Autodesk Inventor part; units mm, degrees
ref_plane "YZ Plane" through (0, 0, 0) normal (1, 0, 0) x (0, 1, 0)
ref_plane "XZ Plane" through (0, 0, 0) normal (0, 1, 0) x (-1, 0, 0)
ref_plane "XY Plane" through (0, 0, 0) normal (0, 0, 1) x (1, 0, 0)
sketch "Skizze1" plane through (0, 0, 0) normal (0, 0, 1) x (1, 0, 0)
  line L0 (0, 0) -> (-67, 0)
  line L1 (-51, 5) -> (0, 5)
  line L2 (0, 5) -> (0, 0)
  line L3 (-51, 5) -> (-51, 2)
  line L4 (-51, 2) -> (-55, 2)
  line L5 (-55, 2) -> (-55, 0)
  line L6 (-56, 0) -> (-55, 0)
  dimension "d0" = 51
  dimension "d42" = 10
  dimension "d60" = 4
  dimension "d61" = 4
revolve "Umdrehung1" add sketch "Skizze1" angle 360 about axis through (0, 0, 0) along (-1, 0, 0)
sketch "Skizze3" plane through (0, 0, 0) normal (0, 1, 0) x (-1, 0, 0)
  line L0 (51, 5) -> (51, -5) construction
  line L1 (51, -5) -> (0, -5) construction
  line L2 (51, 5) -> (0, 5) construction
  line L3 (51, -5) -> (4, -5)
  line L4 (4, -5) -> (4, -3.5)
  line L5 (4, -3.5) -> (51, -3.5)
  line L6 (51, -3.5) -> (51, -5)
  line L7 (4, 5) -> (51, 5)
  line L8 (51, 5) -> (51, 3.5)
  line L9 (51, 3.5) -> (4, 3.5)
  line L10 (4, 3.5) -> (4, 5)
  line L11 (0, 5) -> (0, -5)
  point P0 (0, 0)
  dimension "d10" = 7
  dimension "d11" = 4
extrude "Extrusion1" cut sketch "Skizze3" along normal through all both and the other way through all
sketch "Skizze8" plane through (-4, -3.5707, 3.5) normal (0, 0, 1) x (1, 0, 0)
  line L0 (0, 0) -> (-47, 0) construction
  line L1 (0, 7.1414) -> (0, 0) construction
  line L2 (-47, 7.1414) -> (0, 7.1414) construction
  line L3 (-47, 0) -> (-47, 7.1414) construction
  line L4 (4, -1.4293) -> (4, 8.5707) construction
  point P0 (-39, 3.5707)
  point P1 (4, 3.5707)
  dimension "d63" = 8
hole "Bohrung3" at (-43, 0, 3.5) direction (0, 0, -1) diameter 4 end through all
sketch "Skizze9" plane through (0, 0, 0) normal (1, 0, 0) x (0, 0, -1)
  circle A0 centre (0, 0) radius 5 construction
hole "Bohrung5" at (0, 0, 0) direction (-1, 0, 0) diameter 4.917 depth 12 tip angle 118
properties part number "Shaft_newtest" material "Aluminium 6061"
Here's how the part is built. I have some questions about the finished solid (model axes, mm). A direction names the side the tool comes from. Give positions to 0.01 mm unless a question says otherwise; leave off trailing zeros. Write each loop counter-clockwise with the first axis right and the second up, starting at its lowest first coordinate (ties: lowest second). Pieces come first, ordered by that corner, then holes.
(1) Imagine slicing it at D-D, the plane z = 4. Write out the boundary of the cut face in (x, y).
Output values:
outline: (-4, -3) - (0, -3) - (0, 3) - (-4, 3) - close
(2) Imagine slicing it at A-A, the plane x = -43. Write out the boundary of the cut face in (y, z).
Output values:
outline: (-3.57, -3.5) - (-2, -3.5) - (-2, 3.5) - (-3.57, 3.5) arc R5 ccw to start; (2, -3.5) - (3.57, -3.5) arc R5 ccw to (3.57, 3.5) - (2, 3.5) - close
(3) On a 3-axis mill with a long thin cutter (end or side, diameter ignored), from which of +Z, -Z, +X, -X, +Y, -Y can I reach the whole of each face in a straight line? I mean faces 4 (the face through (-4, 0, 4)), 5 (the face through (-41, 0, 0)), 6 (the face through (-53, 0, 2)), 7 (the face through (-27, 0, -3.5)), 8 (the face through (0, 2, 2)). Say none if no direction works.
Output values:
face 4: +Z, -X, +Y, -Y
face 5: +Z, -Z
face 6: -X
face 7: -Z, -X, +Y, -Y
face 8: +Z, -Z, +X, +Y, -Y
(4) If I drill on L1, parallel to Z at x = -3, y = 0; L2, parallel to Z at x = -5.5, y = 0, over which ranges is the centre line in solid material (lowest first)?
Output values:
L1: z = -5 to -2.46, 2.46 to 5
L2: z = -3.5 to -2.46, 2.46 to 3.5
(5) Thinking about a two-plate mould opening in Z: for faces 1 (the face through (-25, -5, 0)), 2 (the face through (-55, 0, 0)), 3 (the face through (-6.084, -0.738, -2.345)), which applies, pulls with the +Z half, pulls with the -Z half, needs draft (parallel to the pull), parting line crosses it, or undercut?
Output values:
face 1: parting line crosses it
face 2: needs draft
face 3: undercut
(6) Will these pins go through, and if not, where does the flat tip stop? pin 1 (1.5 mm diameter, centred on y = -3.5, z = -1, fed in from -X); pin 2 (1.2 mm diameter, centred on y = 1.5, z = 4.5, fed in from -X); pin 3 (1.5 mm diameter, centred on y = 2, z = 3, fed in from +X); pin 4 (2 mm diameter, centred on x = -22.5, y = 0, fed in from +Z).
Output values:
pin 1: stops at x = -51
pin 2: stops at x = -4
pin 3: stops at x = 0
pin 4: stops at z = 3.5
(7) Imagine slicing it at B-B, the plane z = -3. Write out the boundary of the cut face in (x, y).
Output values:
outline: (-51, -4) - (0, -4) - (0, 4) - (-51, 4) - close; hole circle Ø4 at (-43, 0)
(8) Imagine slicing it at C-C, the plane x = -7. Write out the boundary of the cut face in (y, z).
Output values:
outline: (-3.57, -3.5) - (3.57, -3.5) arc R5 ccw to (3.57, 3.5) - (-3.57, 3.5) arc R5 ccw to start; hole circle Ø4.92 at (0, 0)
